from build123d import *

# Parameters (mm, degrees)
SKETCH1_W                     = 10.16
SKETCH1_H                     = 3.175
SKETCH1_W_2                   = 152.4
SKETCH1_H_2                   = 82.55
SKETCH1_R                     = 7.747
MAIN_EXTRUDE_DEPTH            = 3.175
SKETCH2_R                     = 2.54
CASTER_MOUNTING_HOLES_DEPTH   = 89.274136218
SKETCH3_W                     = 2.54
SKETCH3_H                     = 82.55
REMOVE_UNEVEN_BACK_EDGE_DEPTH = 89.274136218
CUT_EXTRUDE2_DEPTH            = 89.274136218


with BuildPart() as part:
    # Sketch1 → Main Extrude (new body)
    # profile 1 of 7: a face of its own
    with BuildSketch(Plane(origin=(0, 0, 0), x_dir=(1, 0, 0), z_dir=(0, 1, 0))):
        with Locations((43.18, -42.8625)):
            Rectangle(SKETCH1_W, SKETCH1_H)
    # profile 2 of 7: a face of its own
    with BuildSketch(Plane(origin=(0, 0, 0), x_dir=(1, 0, 0), z_dir=(0, 1, 0))):
        Rectangle(SKETCH1_W_2, SKETCH1_H_2)
        with Locations(Location((-65.076590574, 0, 0), (0, 0, 270))):
            Circle(SKETCH1_R, mode=Mode.SUBTRACT)
    # profile 3 of 7: a face of its own
    with BuildSketch(Plane(origin=(0, 0, 0), x_dir=(1, 0, 0), z_dir=(0, 1, 0))):
        with Locations((63.5, -42.8625)):
            Rectangle(SKETCH1_W, SKETCH1_H)
    # profile 4 of 7: a face of its own
    with BuildSketch(Plane(origin=(0, 0, 0), x_dir=(1, 0, 0), z_dir=(0, 1, 0))):
        with Locations((22.86, -42.8625)):
            Rectangle(SKETCH1_W, SKETCH1_H)
    # profile 5 of 7: a face of its own
    with BuildSketch(Plane(origin=(0, 0, 0), x_dir=(1, 0, 0), z_dir=(0, 1, 0))):
        with Locations((63.5, 42.8625)):
            Rectangle(SKETCH1_W, SKETCH1_H)
    # profile 6 of 7: a face of its own
    with BuildSketch(Plane(origin=(0, 0, 0), x_dir=(1, 0, 0), z_dir=(0, 1, 0))):
        with Locations((43.18, 42.8625)):
            Rectangle(SKETCH1_W, SKETCH1_H)
    # profile 7 of 7: a face of its own
    with BuildSketch(Plane(origin=(0, 0, 0), x_dir=(1, 0, 0), z_dir=(0, 1, 0))):
        with Locations((22.86, 42.8625)):
            Rectangle(SKETCH1_W, SKETCH1_H)
    extrude(amount=MAIN_EXTRUDE_DEPTH)

    # Sketch2 → Caster Mounting Holes (cut, through all)
    with BuildSketch(Plane(origin=(0, 3.175, 0), x_dir=(1, 0, 0), z_dir=(0, 1, 0))):
        with Locations(Location((-47.3754273, 15.24, 0), (0, 0, 270))):
            Circle(SKETCH2_R)
        with Locations(Location((-23.4994273, 15.24, 0), (0, 0, 270))):
            Circle(SKETCH2_R)
        with Locations(Location((-23.4994273, -15.24, 0), (0, 0, 270))):
            Circle(SKETCH2_R)
        with Locations(Location((-47.3754273, -15.24, 0), (0, 0, 270))):
            Circle(SKETCH2_R)
    extrude(amount=-CASTER_MOUNTING_HOLES_DEPTH, mode=Mode.SUBTRACT)

    # Sketch3 → Remove Uneven Back Edge (cut, through all)
    with BuildSketch(Plane(origin=(0, 3.175, 0), x_dir=(1, 0, 0), z_dir=(0, 1, 0))):
        with Locations((74.93, 0)):
            Rectangle(SKETCH3_W, SKETCH3_H)
    extrude(amount=-REMOVE_UNEVEN_BACK_EDGE_DEPTH, mode=Mode.SUBTRACT)

    # Sketch4 → Cut-Extrude2 (cut, through all)
    with BuildSketch(Plane(origin=(0, 3.175, 0), x_dir=(1, 0, 0), z_dir=(0, 1, 0))):
        Polygon((12.722439957, 54.007099157), (12.722439957, 28.534320342), (84.718317581, 28.534320342), (84.718317581, -50.041057477), (-114.731091279, -51.937564591), (-115.738488642, 54.007099157), align=None)
    extrude(amount=-CUT_EXTRUDE2_DEPTH, mode=Mode.SUBTRACT)


solid = part.part
Part model, mm, in its own coordinate system. A direction names the side the tool comes from. Coordinates: 2 decimals unless noted, no trailing zeros. Loops run counter-clockwise (first coordinate to the right, second up) from the corner with the lowest first, then second, coordinate; pieces in that order, holes last. Notation, with made-up numbers: (5, -21.75) -> (55, -21.75) arc R10 cw to (55, -5.75) -> close; hole circle Ø2 at (-37, -1). An arc over 180 degrees is marked (long way). Use a Markdown table: item, result. Add a question column.
Item 1: Which spindle directions (+Z, -Z, +X, -X, +Y, -Y) get a long thin tool onto all of the face, cutting with end or side? Do faces 1 (the flat face through (71, 2, -41.275)), 2 (the flat face through (15, 2, -41.275)), 3 (the flat face through (33, 2, -41.275)), 4 (the flat face through (73.66, 2, -35)). Say none if no direction does.
Item 2: Band-saw the part on B-B on y = 0.65. Write the cut outline in (x, z) (3 decimals), plus the area to 3 significant figures.
Item 3: Pull direction X, two halves, no side cores. Call faces 5 (the flat face through (68.58, 2, -43)), 6 (the flat face through (43, 2, -44.45)), 7 (the flat face through (53, 2, -41.275)): +X half, -X half, draft (parallel to the pull), parting line (faces both ways), or undercut.
Item 4: Probe probe 1 along X at (y, z) = (1.15, -43.25); probe 2 along Z at (x, y) = (57, 1.25) (3 decimals). List the from-to ranges inside material, lowest first.
Item 5: Flat gauge pins, fed straight in: P1, Ø1.6, axis at y = 1, z = -43, coming from the -X side; P2, Ø1, axis at y = 1.5, z = -42, coming from the +X side. Where does each tip first touch, or does it go through?
Item 6: Band-saw the part on A-A on z = -42.25. Write the cut outline in (x, y) (3 decimals), plus the area to 3 significant figures.
Item 7: Band-saw the part on C-C on x = 52. Write the cut outline in (y, z) (3 decimals), plus the area to 3 significant figures.
Geometry says:
| question | item | result |
|---|---|---|
| 1 | face 1 | -Z, +X, +Y, -Y |
| 1 | face 2 | -Z, -X, +Y, -Y |
| 1 | face 3 | -Z, +Y, -Y |
| 1 | face 4 | +Z, -Z, +X, +Y, -Y |
| 2 | outline | (12.722, -41.275) -> (17.78, -41.275) -> (17.78, -44.45) -> (27.94, -44.45) -> (27.94, -41.275) -> (38.1, -41.275) -> (38.1, -44.45) -> (48.26, -44.45) -> (48.26, -41.275) -> (58.42, -41.275) -> (58.42, -44.45) -> (68.58, -44.45) -> (68.58, -41.275) -> (73.66, -41.275) -> (73.66, -28.534) -> (12.722, -28.534) -> close |
| 2 | area | 873 mm² |
| 3 | face 5 | +X half |
| 3 | face 6 | draft |
| 3 | face 7 | undercut |
| 4 | probe 1 | 17.78 to 27.94, 38.1 to 48.26, 58.42 to 68.58 |
| 4 | probe 2 | -41.275 to -28.534 |
| 5 | P1 | x = 17.78 |
| 5 | P2 | x = 68.58 |
| 6 | outline | (17.78, 0) -> (27.94, 0) -> (27.94, 3.175) -> (17.78, 3.175) -> close; (38.1, 0) -> (48.26, 0) -> (48.26, 3.175) -> (38.1, 3.175) -> close; (58.42, 0) -> (68.58, 0) -> (68.58, 3.175) -> (58.42, 3.175) -> close |
| 6 | area | 96.8 mm² |
| 7 | outline | (0, -41.275) -> (3.175, -41.275) -> (3.175, -28.534) -> (0, -28.534) -> close |
| 7 | area | 40.5 mm² |
